Read the model definition and answer for the solid it produces. Units are mm, in the model's axes. Coordinates: 2 decimals unless noted, no trailing zeros. Loops run counter-clockwise (first coordinate to the right, second up) from the corner with the lowest first, then second, coordinate; pieces in that order, holes last.
from build123d import *

# Parameters (mm, degrees)
F0_R     = 1.27
F0_R_2   = 5.969
F0_R_3   = 2.54
F1_DEPTH = 3.1242


with BuildPart() as f1:
    # F0 (on Front) → F1 (new body)
    with BuildSketch(Plane.XZ):
        with BuildLine():
            ThreePointArc((-18.415, 0), (0, -18.415), (18.415, 0))
            ThreePointArc((18.415, 0), (13.021371, 13.021371), (0, 18.415))
            ThreePointArc((0, 18.415), (-13.021371, 13.021371), (-18.415, 0))
        make_face()
        with Locations((-7.62, -13.198227)):
            Circle(F0_R, mode=Mode.SUBTRACT)
        with Locations((-15.24, 0)):
            Circle(F0_R, mode=Mode.SUBTRACT)
        with Locations((7.62, -13.198227)):
            Circle(F0_R, mode=Mode.SUBTRACT)
        with Locations((15.24, 0)):
            Circle(F0_R, mode=Mode.SUBTRACT)
        with Locations((-7.62, 13.198227)):
            Circle(F0_R, mode=Mode.SUBTRACT)
        with Locations((0, 7.366)):
            Circle(F0_R_2, mode=Mode.SUBTRACT)
        with Locations((7.62, 13.198227)):
            Circle(F0_R, mode=Mode.SUBTRACT)
        with BuildLine():
            ThreePointArc((-18.415, 0), (-13.021371, 13.021371), (0, 18.415))
            Line((0, 18.415), (-42.277626, 18.415))
            Line((-42.277626, 18.415), (-42.277626, 0))
            Line((-42.277626, 0), (-18.415, 0))
        make_face()
        with Locations((-29.577626, 7.366)):
            Circle(F0_R_3, mode=Mode.SUBTRACT)
        with BuildLine():
            ThreePointArc((0, 18.415), (13.021371, 13.021371), (18.415, 0))
            Line((18.415, 0), (42.277626, 0))
            Line((42.277626, 0), (42.277626, 18.415))
            Line((42.277626, 18.415), (0, 18.415))
        make_face()
        with Locations((29.577626, 7.366)):
            Circle(F0_R_3, mode=Mode.SUBTRACT)
    extrude(amount=F1_DEPTH)


solid = f1.part
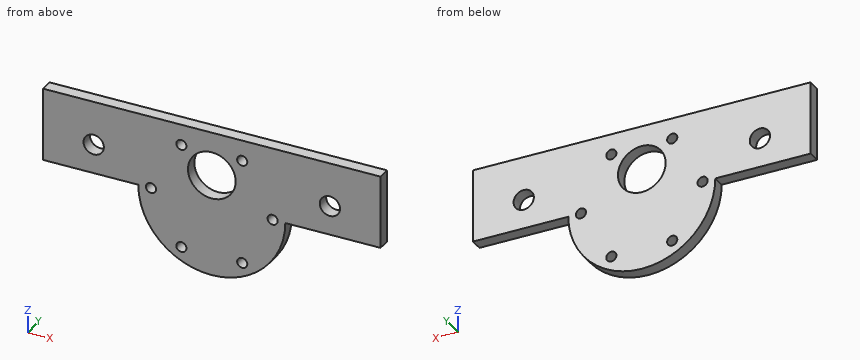
Q1. A flat-ended cylindrical pin translates along its axis: pin 1 Ø1.6 at (x, y) = (25, -2) entering from -Z. Find the tip coordinate at first contact, or state that the pin passes through.
Findings below:
pin 1: stops at z = 0
Q2. A cutting plane is placed at B-B (y = -1.75). Count the separate pieces of the cut face and the enclosed holes in it, then the cut area to 3 significant figures.
Findings below:
separate pieces: 1
enclosed holes: 9
area: 1,910 mm2
Q3. A cutting plane is placed at C-C (z = 6.5). Give the vertices of the cut face in (x, y), then the cut area to 3 significant figures.
Findings below:
outline: (-42.28, -3.12) - (-31.97, -3.12) - (-31.97, 0) - (-42.28, 0) - close; (-27.19, -3.12) - (-5.91, -3.12) - (-5.91, 0) - (-27.19, 0) - close; (5.91, -3.12) - (27.19, -3.12) - (27.19, 0) - (5.91, 0) - close; (31.97, -3.12) - (42.28, -3.12) - (42.28, 0) - (31.97, 0) - close
area: 197 mm2
Q4. A cutting plane is placed at D-D (x = -28). Give the vertices of the cut face in (y, z) (3 decimals).
Findings below:
outline: (-3.124, 0) - (0, 0) - (0, 5.375) - (-3.124, 5.375) - close; (-3.124, 9.357) - (0, 9.357) - (0, 18.415) - (-3.124, 18.415) - close
Q5. A cutting plane is placed at A-A (x = 0). Give the vertices of the cut face in (y, z) (3 decimals), then the cut area to 3 significant figures.
Findings below:
outline: (-3.124, -18.415) - (0, -18.415) - (0, 1.397) - (-3.124, 1.397) - close; (-3.124, 13.335) - (0, 13.335) - (0, 18.415) - (-3.124, 18.415) - close
area: 77.8 mm2
Q6. Straight lines are drawn through the part: probe 1 along Z at (x, y) = (7, -1.9) (3 decimals); probe 2 along Z at (x, y) = (-7.62, -2.05) (3 decimals); probe 3 along X at (y, z) = (-2.7, -14). For each, find the intervals that lie inside material, in ascending order.
Findings below:
probe 1: z = -17.033 to -14.307, -12.09 to 12.09, 14.307 to 18.415
probe 2: z = -16.764 to -14.468, -11.928 to 11.928, 14.468 to 18.415
probe 3: x = -11.96 to -8.6, -6.64 to 6.64, 8.6 to 11.96
